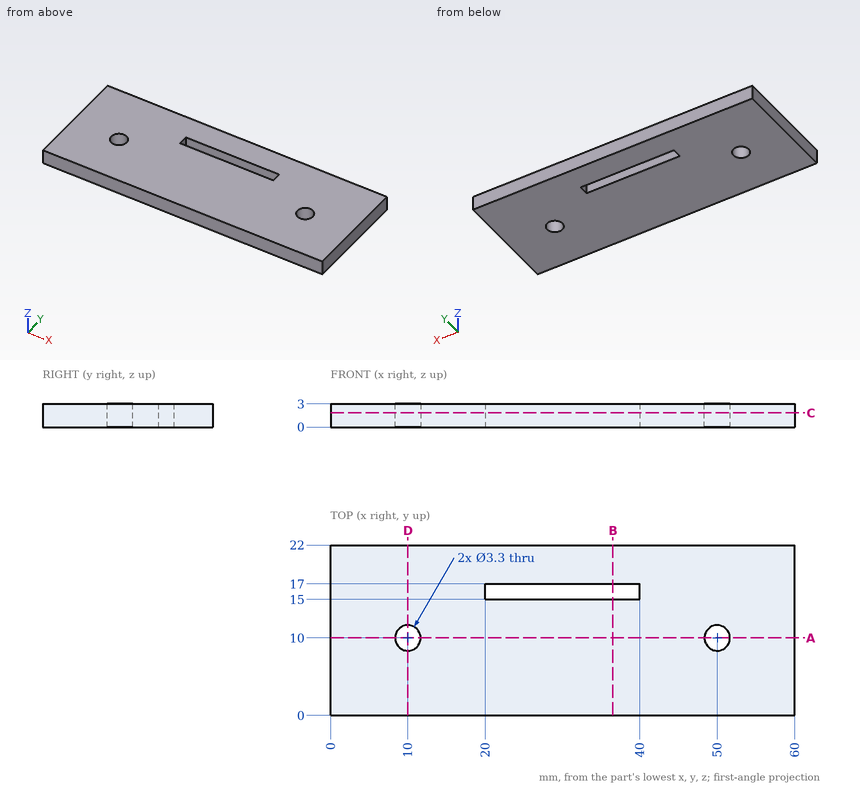
Source: three-view drawing plus pictorial views. Frame: mm from the lowest corner of the part. Round coordinates to 2 decimals unless told otherwise and drop trailing zeros. Loops run counter-clockwise (first coordinate to the right, second up) from the corner with the lowest first, then second, coordinate; pieces in that order, holes last.
1. Section query A-A on y = 10. Output: boundary loops of the cut face in (x, z).
2. Ray query, L1, parallel to X at y = 15.75, z = 2.35; L2, parallel to Y at x = 10, z = 1; L3, parallel to X at y = 11.25, z = 1.3. Return the intervals inside material, ascending.
3. Section query D-D on x = 10. Output: boundary loops of the cut face in (y, z), and give its area (3 significant figures).
4. Section query B-B on x = 36.5. Output: boundary loops of the cut face in (y, z), and give its area (3 significant figures).
5. Section query C-C on z = 1.85. Output: boundary loops of the cut face in (x, y), and give its area (3 significant figures).
Answers below:
1. outline: (0, 0) - (8.35, 0) - (8.35, 3) - (0, 3) - close; (11.65, 0) - (48.35, 0) - (48.35, 3) - (11.65, 3) - close; (51.65, 0) - (60, 0) - (60, 3) - (51.65, 3) - close
2. L1: x = 0 to 20, 40 to 60
2. L2: y = 0 to 8.35, 11.65 to 22
2. L3: x = 0 to 8.92, 11.08 to 48.92, 51.08 to 60
3. outline: (0, 0) - (8.35, 0) - (8.35, 3) - (0, 3) - close; (11.65, 0) - (22, 0) - (22, 3) - (11.65, 3) - close
3. area: 56.1 mm2
4. outline: (0, 0) - (15, 0) - (15, 3) - (0, 3) - close; (17, 0) - (22, 0) - (22, 3) - (17, 3) - close
4. area: 60.0 mm2
5. outline: (0, 0) - (60, 0) - (60, 22) - (0, 22) - close; hole circle Ø3.3 at (10, 10); hole (20, 15) - (40, 15) - (40, 17) - (20, 17) - close; hole circle Ø3.3 at (50, 10)
5. area: 1,260 mm2
